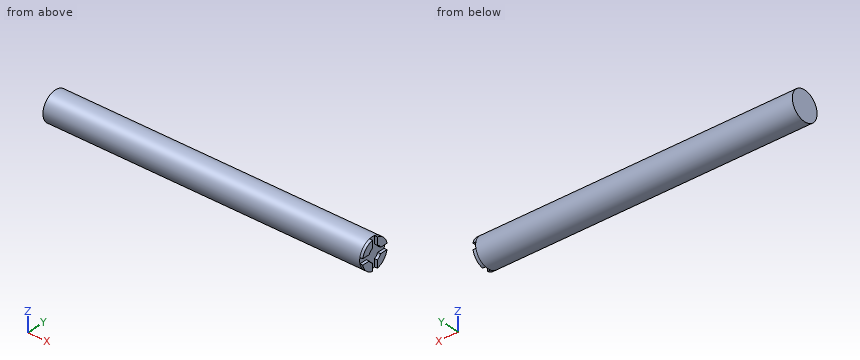
from build123d import *

# Parameters (mm, degrees)
F0_R     = 12.7
F1_DEPTH = 276.86
F3_DEPTH = 2.54


# Not quite as in the source:
# - after a boolean that leaves OpenCascade's solid faulty, fix() repairs it


with BuildPart() as f1:
    # F0 (on Right) → F1 (new body)
    with BuildSketch(Plane.YZ):
        Circle(F0_R)
    extrude(amount=-F1_DEPTH)

    # F2 (on face) → F3 (join)
    with BuildSketch(Plane.YZ):
        with BuildLine():
            ThreePointArc((-5.8198711326, 2.54), (-4.4901280605, 4.4901280605), (-2.54, 5.8198711326))
            Line((-2.54, 5.8198711326), (-2.54, 12.4434078933))
            ThreePointArc((-2.54, 12.4434078933), (-8.9802561211, 8.9802561211), (-12.4434078933, 2.54))
            Line((-12.4434078933, 2.54), (-5.8198711326, 2.54))
        make_face()
        with BuildLine():
            ThreePointArc((2.54, 5.8198711326), (4.4901280605, 4.4901280605), (5.8198711326, 2.54))
            Line((5.8198711326, 2.54), (12.4434078933, 2.54))
            ThreePointArc((12.4434078933, 2.54), (8.9802561211, 8.9802561211), (2.54, 12.4434078933))
            Line((2.54, 12.4434078933), (2.54, 5.8198711326))
        make_face()
        with BuildLine():
            Line((12.4434078933, -2.54), (5.8198711326, -2.54))
            ThreePointArc((5.8198711326, -2.54), (4.4901280605, -4.4901280605), (2.54, -5.8198711326))
            Line((2.54, -5.8198711326), (2.54, -12.4434078933))
            ThreePointArc((2.54, -12.4434078933), (8.9802561211, -8.9802561211), (12.4434078933, -2.54))
        make_face()
        with BuildLine():
            Line((-2.54, -12.4434078933), (-2.54, -5.8198711326))
            ThreePointArc((-2.54, -5.8198711326), (-4.4901280605, -4.4901280605), (-5.8198711326, -2.54))
            Line((-5.8198711326, -2.54), (-12.4434078933, -2.54))
            ThreePointArc((-12.4434078933, -2.54), (-8.9802561211, -8.9802561211), (-2.54, -12.4434078933))
        make_face()
    extrude(amount=F3_DEPTH)

    add(f1.part.fix(), mode=Mode.REPLACE)


solid = f1.part
The listing builds one solid part. Answer for the finished solid, in the listing's coordinates (mm). Round coordinates to 2 decimals unless told otherwise and drop trailing zeros. Write each loop counter-clockwise with the first axis right and the second up, starting at its lowest first coordinate (ties: lowest second). Pieces come first, ordered by that corner, then holes. Notation, with made-up numbers: (48.5, 25.25) - (103.5, 25.25) arc R14 ccw to (103.5, 46.25) - close; hole circle Ø1 at (45, 57.5). An arc over 180 degrees is marked (long way). Use a Markdown table: item, result. Add a question column.
1. The part is cut by section B-B (y = 9.25). Write down the section's boundary in (x, z).
2. Consider line 1 (X direction, y = -1.25, z = -4); line 2 (Y direction, x = -84, z = 2.25); line 3 (Y direction, x = -221.5, z = 2.75). Determine where each line is inside the solid, lowest interval first.
3. The part is cut by section A-A (z = -10). Write down the section's boundary in (x, y).
4. Flat-ended cylindrical pins translate along their axes: P1, Ø0.8, axis at x = 1.5, y = -7.5, coming from the +Z side; P2, Ø2, axis at x = 1.5, z = 9, coming from the -Y side; P3, Ø3, axis at x = 1, y = 10.5, coming from the +Z side. Find the tip coordinate at first contact, or state that the pin passes through.
5. The part is cut by section C-C (x = -115). Write down the section's boundary in (y, z), and give its area (3 significant figures).
Reported:
| question | item | result |
|---|---|---|
| 1 | outline | (-276.86, -8.7) - (2.54, -8.7) - (2.54, -2.54) - (0, -2.54) - (0, 2.54) - (2.54, 2.54) - (2.54, 8.7) - (-276.86, 8.7) - close |
| 2 | line 1 | -276.86 to 0 |
| 2 | line 2 | -12.5 to 12.5 |
| 2 | line 3 | -12.4 to 12.4 |
| 3 | outline | (-276.86, -7.83) - (2.54, -7.83) - (2.54, -2.54) - (0, -2.54) - (0, 2.54) - (2.54, 2.54) - (2.54, 7.83) - (-276.86, 7.83) - close |
| 4 | P1 | z = 10.53 |
| 4 | P2 | y = -9.86 |
| 4 | P3 | z = 8.96 |
| 5 | outline | circle Ø25.4 at (0, 0) |
| 5 | area | 507 mm^2 |
